```python
from build123d import *

# Parameters (mm, degrees)
SKETCH133_R          = 2.15
PAD070_DEPTH         = 3
PAD071_DEPTH         = 8
SKETCH135_R          = 25.5
POCKET019_DEPTH      = 17.388212
POCKET019_DEPTH_BACK = 14.320967
CHAMFER011_SIZE2     = 7
CHAMFER011_SIZE      = 9
SKETCH136_R          = 5
POCKET020_DEPTH      = 14.001
FILLET011_R          = 6
FILLET012_R          = 1
SKETCH137_W          = 12
SKETCH137_H          = 4
PAD072_DEPTH         = 4


with BuildPart() as part:
    # Sketch133 → Pad070 (new body)
    with BuildSketch(Plane.XY):
        Polygon((12, -6), (12, 6), (-12, 6), (-12, -6), (-12, -8), (12, -8), align=None)
        with Locations((6, 0)):
            Circle(SKETCH133_R, mode=Mode.SUBTRACT)
        with Locations((-6, 0)):
            Circle(SKETCH133_R, mode=Mode.SUBTRACT)
    extrude(amount=PAD070_DEPTH)

    # Sketch134 → Pad071 (join, symmetric)
    with BuildSketch(Plane.YZ):
        Polygon((-4, 3), (-8, 3), (-8, 4), (-30, 4), (-30, 7.4), (-25, 17), (-4, 17), align=None)
    extrude(amount=PAD071_DEPTH, both=True)

    # Sketch135 (on DatumPlane) → Pocket019 (cut, two sides)
    with BuildSketch(Plane(origin=(8, -25, 17), x_dir=(-1, 0, 0), z_dir=(0, 0.461934, 0.886914))) as pocket019_sk:
        with Locations((8, 23)):
            Circle(SKETCH135_R)
    extrude(amount=-POCKET019_DEPTH, mode=Mode.SUBTRACT)
    extrude(pocket019_sk.sketch, amount=POCKET019_DEPTH_BACK, mode=Mode.SUBTRACT)

    # Chamfer011
    chamfer011_edges = [part.edges().sort_by_distance(p)[0] for p in [
        (0, -4, 17),
    ]]
    chamfer011_side = part.faces().sort_by_distance((0, -4, 10))[0]
    chamfer(chamfer011_edges, length=CHAMFER011_SIZE, length2=CHAMFER011_SIZE2, reference=chamfer011_side)

    # Sketch136 (on Face7 of Chamfer011) → Pocket020 (cut, through all)
    with BuildSketch(Plane.XY.offset(3)):
        with Locations((-6, 0)):
            Circle(SKETCH136_R)
        with Locations((6, 0)):
            Circle(SKETCH136_R)
    extrude(amount=POCKET020_DEPTH, mode=Mode.SUBTRACT)

    # Fillet011
    fillet011_edges = [part.edges().sort_by_distance(p)[0] for p in [
        (-12, 6, 1.5),
        (12, 6, 1.5),
    ]]
    fillet(fillet011_edges, radius=FILLET011_R)

    # Fillet012
    fillet012_edges = [part.edges().sort_by_distance(p)[0] for p in [
        (0, -22.181238, 17),
        (0, -28.952071, 4),
    ]]
    fillet(fillet012_edges, radius=FILLET012_R)

    # Sketch137 (on Face2 of Fillet012) → Pad072 (join)
    with BuildSketch(Plane(origin=(0, 0, 4), x_dir=(1, 0, 0), z_dir=(0, 0, -1))):
        with Locations((0, 16.4)):
            Rectangle(SKETCH137_W, SKETCH137_H)
    extrude(amount=PAD072_DEPTH)


with BuildPart() as part_1:
    # Body031 placement: moved
    add(part.part.moved(Location((0, 33.5, -181.5))))


solid = part_1.part
```
Check sheet for the modelled part. Datum: model origin and axes. Units: mm. A direction names the side the tool comes from. Round coordinates to 2 decimals unless told otherwise and drop trailing zeros. Loops run counter-clockwise (first coordinate to the right, second up) from the corner with the lowest first, then second, coordinate; pieces in that order, holes last. Notation, with made-up numbers: M -13,-13.5 L 46,-13.5 A13 cw 46,-9.5 Z; hole C -36.75,-1 d6. An arc over 180 degrees is marked long. Answer as a JSON object with one key per item and string values.
1. Mould release check, pull along Y, two halves, no side actions. Record for faces 1 (the cylindrical face through (-6.28, 35.63, -180.02)), 2 (the flat face through (-6, 17, -179)), 3 (the cylindrical face through (-10.289, 37.696, -179.979)): pulls with the +Y half, pulls with the -Y half, needs draft (parallel to the pull), parting line crosses it, or undercut.
Reply:
{"face 1": "undercut", "face 2": "needs draft", "face 3": "pulls with the +Y half"}
2. Section check B-B (y = 23). Record the boundary of the cut face in (x, z), plus the area to 3 significant figures.
Reply:
{"outline": "M -8,-177.5 L 8,-177.5 L 8,-165.14 L -8,-165.14 Z", "area": "198 mm²"}
3. Section check A-A (y = 12.5). Record the boundary of the cut face in (x, z).
Reply:
{"outline": "M -8,-177.5 L 8,-177.5 L 8,-164.5 L -8,-164.5 Z"}
4. Scan lines: line 1 (Z direction, x = 1.5, y = 21); line 2 (Z direction, x = -1, y = 34); line 3 (Y direction, x = -2.5, z = -179.75). Record each from-to range of solid material in increasing order.
Reply:
{"line 1": "z = -177.5 to -164.5", "line 2": "z = -181.5 to -178.5", "line 3": "y = 15.1 to 19.1, 25.5 to 39.5"}
5. Access from +Z, -Z, +X, -X, +Y, -Y to the whole of each face (thin tool, end or side, straight path). Record for faces 4 (the flat face through (12, 29, -180)), 5 (the cylindrical face through (-5.46, 28.53, -175.34)), 6 (the flat face through (0, 15.1, -179)), 7 (the flat face through (0, 19.1, -179)), 8 (the flat face through (0, 17, -181.5)).
Reply:
{"face 4": "+Z, -Z, +X, +Y, -Y", "face 5": "+Z, +Y", "face 6": "-Z, +X, -X, -Y", "face 7": "-Z, +X, -X", "face 8": "-Z, +X, -X, +Y, -Y"}
6. Gauge pin test, flat ends, axial feed: P1, Ø2, axis at x = 4, z = -179.5, coming from the -Y side; P2, Ø4.5, axis at y = 17, z = -180, coming from the -X side; P3, Ø2, axis at x = 9.5, z = -171, coming from the +Y side; P4, Ø2.5, axis at x = 1.5, z = -175.5, coming from the +Y side. Record the tip position at first contact, or that the pin passes through.
Reply:
{"P1": "stops at y = 15.1", "P2": "stops at x = -6", "P3": "passes through", "P4": "stops at y = 29.5"}
